Geometry: see drawing. Coordinates: mm, zero at the bounding-box minimum. A direction names the side the tool comes from. Coordinates: 2 decimals unless noted, no trailing zeros. Loops run counter-clockwise (first coordinate to the right, second up) from the corner with the lowest first, then second, coordinate; pieces in that order, holes last. Notation, with made-up numbers: (32, -17.75) - (59, -17.75) arc R29 ccw to (59, 13.25) - close; hole circle Ø2 at (31, -30.75). An arc over 180 degrees is marked (long way). Answer in a Markdown table with one row per item.
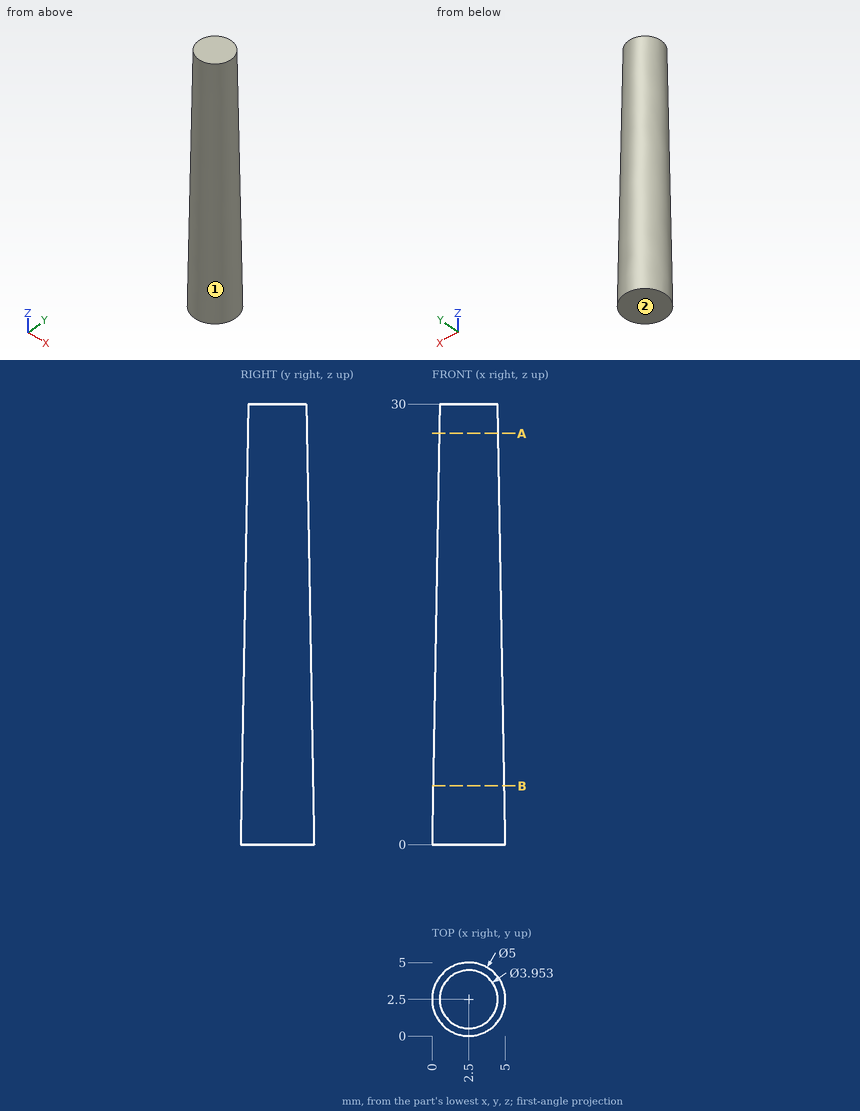
(1) First-contact query: pin 1 Ø3 at (x, z) = (1, 10.5) entering from +Y; pin 2 Ø1.5 at (y, z) = (1, 5) entering from -X; pin 3 Ø2 at (y, z) = (3, 20.5) entering from -X. Flat tips, straight axial feed; report the tip coordinate or a pass-through.
Verdict:
| item | result |
|---|---|
| pin 1 | stops at y = 4.82 |
| pin 2 | stops at x = 0.21 |
| pin 3 | stops at x = 0.34 |
(2) Access query for the marked faces 1 and 2. Directions: +Z, -Z, +X, -X, +Y, -Y. A direction counts if a zero-diameter tool reaches every point of the face in a straight line with its end or side. Return the directions, or none.
Verdict:
| item | result |
|---|---|
| face 1 | +Z |
| face 2 | -Z, +X, -X, +Y, -Y |
(3) Cut plane A-A on z = 28. Output: boundary loops of the cut face in (x, y), then the cut area to 3 significant figures.
Verdict:
| item | result |
|---|---|
| outline | circle Ø4.02 at (2.5, 2.5) |
| area | 12.7 mm² |
(4) Cut plane B-B on z = 4. Output: boundary loops of the cut face in (x, y).
Verdict:
| item | result |
|---|---|
| outline | circle Ø4.86 at (2.5, 2.5) |
(5) Ray query, probe 1 along X at (y, z) = (0.8, 8.5) (1 decimal); probe 2 along Y at (x, z) = (2.45, 6) (1 decimal); probe 3 along X at (y, z) = (2.4, 18). Return the intervals inside material, ascending.
Verdict:
| item | result |
|---|---|
| probe 1 | x = 0.9 to 4.1 |
| probe 2 | y = 0.1 to 4.9 |
| probe 3 | x = 0.32 to 4.68 |
